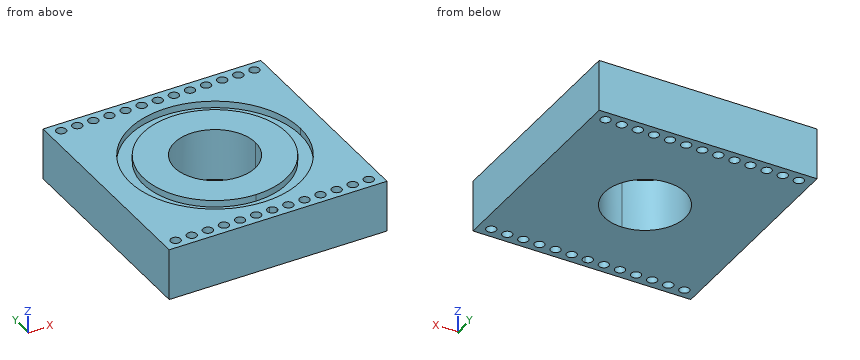
```python
from build123d import *

# Parameters (mm, degrees)
F0_R     = 11
F1_DEPTH = 115
F2_DEPTH = 115
F3_DEPTH = 100


with BuildPart() as f1:
    # F0 (on Top) → F1 (new body)
    with BuildSketch(Plane.XY):
        Polygon((0, -245), (242.5, -245), (242.5, 245), (-242.5, 245), (-242.5, -245), align=None)
        with Locations((-215.1, -222.25)):
            Circle(F0_R, mode=Mode.SUBTRACT)
        with Locations((-179.25, -222.25)):
            Circle(F0_R, mode=Mode.SUBTRACT)
        with Locations((-143.4, -222.25)):
            Circle(F0_R, mode=Mode.SUBTRACT)
        with Locations((-107.55, -222.25)):
            Circle(F0_R, mode=Mode.SUBTRACT)
        with Locations((-71.7, -222.25)):
            Circle(F0_R, mode=Mode.SUBTRACT)
        with Locations((-35.85, -222.25)):
            Circle(F0_R, mode=Mode.SUBTRACT)
        with BuildLine():
            ThreePointArc((11, -222.25), (7.778175, -230.028175), (0, -233.25))
            ThreePointArc((0, -233.25), (-11, -222.25), (0, -211.25))
            ThreePointArc((0, -211.25), (7.778175, -214.471825), (11, -222.25))
        make_face(mode=Mode.SUBTRACT)
        with Locations((35.85, -222.25)):
            Circle(F0_R, mode=Mode.SUBTRACT)
        with Locations((71.7, -222.25)):
            Circle(F0_R, mode=Mode.SUBTRACT)
        with Locations((107.55, -222.25)):
            Circle(F0_R, mode=Mode.SUBTRACT)
        with Locations((143.4, -222.215042)):
            Circle(F0_R, mode=Mode.SUBTRACT)
        with Locations((179.25, -222.215042)):
            Circle(F0_R, mode=Mode.SUBTRACT)
        with Locations((215.1, -221.956581)):
            Circle(F0_R, mode=Mode.SUBTRACT)
        with Locations((-215.1, 222.25)):
            Circle(F0_R, mode=Mode.SUBTRACT)
        with Locations((-179.25, 222.25)):
            Circle(F0_R, mode=Mode.SUBTRACT)
        with Locations((-143.4, 222.25)):
            Circle(F0_R, mode=Mode.SUBTRACT)
        with Locations((-107.55, 222.25)):
            Circle(F0_R, mode=Mode.SUBTRACT)
        with Locations((-71.7, 222.25)):
            Circle(F0_R, mode=Mode.SUBTRACT)
        with Locations((-35.85, 222.25)):
            Circle(F0_R, mode=Mode.SUBTRACT)
        with BuildLine():
            ThreePointArc((190, 0), (134.350288, -134.350288), (0, -190))
            ThreePointArc((0, -190), (-134.350288, 134.350288), (190, 0))
        make_face(mode=Mode.SUBTRACT)
        with Locations((0, 222.25)):
            Circle(F0_R, mode=Mode.SUBTRACT)
        with Locations((35.85, 222.25)):
            Circle(F0_R, mode=Mode.SUBTRACT)
        with Locations((71.7, 222.25)):
            Circle(F0_R, mode=Mode.SUBTRACT)
        with Locations((107.55, 222.25)):
            Circle(F0_R, mode=Mode.SUBTRACT)
        with Locations((143.4, 222.215042)):
            Circle(F0_R, mode=Mode.SUBTRACT)
        with Locations((179.25, 222.215042)):
            Circle(F0_R, mode=Mode.SUBTRACT)
        with Locations((215.1, 221.956581)):
            Circle(F0_R, mode=Mode.SUBTRACT)
    extrude(amount=F1_DEPTH)



with BuildPart() as f2:
    # F0 (on Top) → F2 (new body)
    with BuildSketch(Plane.XY):
        with BuildLine():
            ThreePointArc((160, 0), (-113.137085, 113.137085), (0, -160))
            ThreePointArc((0, -160), (113.137085, -113.137085), (160, 0))
        make_face()
        with BuildLine():
            ThreePointArc((90, 0), (63.63961, -63.63961), (0, -90))
            ThreePointArc((0, -90), (-63.63961, 63.63961), (90, 0))
        make_face(mode=Mode.SUBTRACT)
    extrude(amount=F2_DEPTH)


with BuildPart() as f1_1:
    add(f1.part)

    add(f2.part)  # F3 merges F2
    # F0 (on Top) → F3 (join)
    with BuildSketch(Plane.XY):
        with BuildLine():
            ThreePointArc((190, 0), (-134.350288, 134.350288), (0, -190))
            ThreePointArc((0, -190), (134.350288, -134.350288), (190, 0))
        make_face()
        with BuildLine():
            ThreePointArc((160, 0), (113.137085, -113.137085), (0, -160))
            ThreePointArc((0, -160), (-113.137085, 113.137085), (160, 0))
        make_face(mode=Mode.SUBTRACT)
    extrude(amount=F3_DEPTH)


solid = f1_1.part
```
Can you work these out from the model? Positions are in its coordinate system, mm. Round coordinates to 2 decimals unless told otherwise and drop trailing zeros. Order: outer loops, then holes, each group sorted by start corner. A loop starts at its lowest first (then second) coordinate and runs counter-clockwise, first axis right, second up.
(1) If we section it at A-A (x = 147): Please give me the cut outline in (y, z), plus the area to 3 significant figures.
Results are:
outline: (-245, 0) - (-232.61, 0) - (-232.61, 115) - (-245, 115) - close; (-211.82, 0) - (211.82, 0) - (211.82, 115) - (120.38, 115) - (120.38, 100) - (63.17, 100) - (63.17, 115) - (-63.17, 115) - (-63.17, 100) - (-120.38, 100) - (-120.38, 115) - (-211.82, 115) - close; (232.61, 0) - (245, 0) - (245, 115) - (232.61, 115) - close
area: 49,900 mm2
(2) If we section it at C-C (x = -77): Please give me the cut outline in (y, z).
Results are:
outline: (-245, 0) - (-231.89, 0) - (-231.89, 115) - (-245, 115) - close; (-212.61, 0) - (-46.59, 0) - (-46.59, 115) - (-140.25, 115) - (-140.25, 100) - (-173.7, 100) - (-173.7, 115) - (-212.61, 115) - close; (46.59, 0) - (212.61, 0) - (212.61, 115) - (173.7, 115) - (173.7, 100) - (140.25, 100) - (140.25, 115) - (46.59, 115) - close; (231.89, 0) - (245, 0) - (245, 115) - (231.89, 115) - close
(3) If we section it at B-B (y = -43): Please give me the cut outline in (x, z).
Results are:
outline: (-242.5, 0) - (-79.06, 0) - (-79.06, 115) - (-154.11, 115) - (-154.11, 100) - (-185.07, 100) - (-185.07, 115) - (-242.5, 115) - close; (79.06, 0) - (242.5, 0) - (242.5, 115) - (185.07, 115) - (185.07, 100) - (154.11, 100) - (154.11, 115) - (79.06, 115) - close
(4) If we section it at D-D (z = 108): Count the separate pieces of the cut face and the enclosed holes in it, plus the area to 3 significant figures.
Results are:
separate pieces: 2
enclosed holes: 28
area: 169,000 mm2
(5) I'm going to push a flat-ended pin straight in: pin 1 (3 mm diameter, centred on x = -107, y = 144, fed in from +Z). Where does the tip first touch, or does it pass through?
Results are:
pin 1: stops at z = 100
(6) If I drill on L1, parallel to Y at x = 107, z = 54; L2, parallel to Y at x = 179, z = 85; L3, parallel to Y at x = 39, z = 57.5, over which ranges is the centre line in solid material (lowest first)?
Results are:
L1: y = -245 to -233.24, -211.26 to 211.26, 233.24 to 245
L2: y = -245 to -233.21, -211.22 to 211.22, 233.21 to 245
L3: y = -245 to -232.79, -211.71 to -81.11, 81.11 to 211.71, 232.79 to 245
